Autodesk Inventor part; units mm, degrees
ref_plane "YZ Plane" through (0, 0, 0) normal (1, 0, 0) x (0, 1, 0)
ref_plane "XZ Plane" through (0, 0, 0) normal (0, 1, 0) x (-1, 0, 0)
ref_plane "XY Plane" through (0, 0, 0) normal (0, 0, 1) x (1, 0, 0)
sketch "Sketch1" plane through (0, 0, 0) normal (0, 0, 1) x (1, 0, 0)
  line L0 (2.4705, -2.1641) -> (-67.5295, -2.1641)
  line L1 (-67.5295, -2.1641) -> (-67.5295, 10.5359)
  line L2 (-67.5295, 10.5359) -> (2.4705, 10.5359)
  line L3 (2.4705, 10.5359) -> (2.4705, -2.1641)
  dimension "d0" = 12.7
  dimension "d1" = 70
extrude "Extrusion1" add sketch "Sketch1" along normal blind 567.2
sketch "Sketch2" plane through (2.4705, -2.1641, 0) normal (1, 0, 0) x (0, 0, -1)
  line L0 (-567.3829, 6.35) -> (0, 6.35) construction
  line L1 (0, 12.7) -> (-567.2, 12.7) construction
  line L2 (-567.2, 12.7) -> (-567.2, 0) construction
  point P0 (-543.6, 6.35)
  point P1 (-33.6, 6.35)
  point P2 (-133.6, 6.35)
  point P3 (-238.6, 6.35)
  point P4 (-338.6, 6.35)
  point P5 (-443.6, 6.35)
  dimension "d4" = 6.35
  dimension "d5" = 23.6
  dimension "d6" = 100
  dimension "d7" = 105
  dimension "d8" = 100
  dimension "d9" = 105
  dimension "d10" = 100
  dimension "d11" = 33.6
  dimension "d12" = 567.3829
hole "Hole1" [suppressed]
sketch "Sketch3" plane through (0, 0, 567.2) normal (0, 0, 1) x (1, 0, 0)
  line L0 (-67.5295, -2.1641) -> (-67.5295, 10.5359)
  line L1 (-67.5295, 10.5359) -> (2.4705, 10.5359)
  line L2 (2.4705, -2.1641) -> (-67.5295, -2.1641)
  line L3 (2.4705, 10.5359) -> (2.4705, -2.1641)
extrude "Extrusion2" add sketch "Sketch3" along normal blind 150
sketch "Sketch4" plane through (0, 0, 0) normal (0, 0, -1) x (-1, 0, 0)
  line L0 (-2.4705, -2.1641) -> (67.5295, -2.1641)
  line L1 (67.5295, -2.1641) -> (67.5295, 10.5359)
  line L2 (67.5295, 10.5359) -> (-2.4705, 10.5359)
  line L3 (-2.4705, 10.5359) -> (-2.4705, -2.1641)
extrude "Extrusion3" add sketch "Sketch4" along normal blind 150
sketch "Sketch5" plane through (2.4705, -2.1641, 717.2) normal (1, 0, 0) x (0, 0, -1)
  circle A0 centre (73.972, 6.35) radius 3.9687
  circle A1 centre (113.972, 6.35) radius 3.9687
  circle A2 centre (748.257, 6.35) radius 3.9687
  circle A3 centre (798.257, 6.35) radius 3.9687
hole "Hole2" [suppressed]
sketch "Sketch6" plane through (2.4705, -2.1641, 717.2) normal (1, 0, 0) x (0, 0, -1)
  line L0 (867.2, 0) -> (0, 0)
  line L1 (0, 12.7) -> (0, 0)
  line L2 (0, 12.7) -> (867.2, 12.7)
  line L3 (63.972, 12.7) -> (63.972, 0)
  line L4 (63.972, 12.7) -> (0, 12.7)
  line L5 (0, 0) -> (63.972, 0)
  line L6 (0, 0) -> (0, 12.7)
  circle A0 centre (73.972, 6.35) radius 3.9687
  dimension "d31" = 10
extrude "Extrusion4" cut sketch "Sketch6" against normal blind 70 contours L0 L1 L2 L3
sketch "Sketch7" plane through (2.4705, -2.1641, 653.228) normal (1, 0, 0) x (0, 0, -1)
  line L0 (803.228, 0) -> (0, 0)
  line L1 (0, 12.7) -> (803.228, 12.7)
  line L2 (803.228, 0) -> (803.228, 12.7)
  circle A0 centre (734.285, 6.35) radius 3.9687
  line L3 (749.285, 12.7) -> (749.285, 0)
  line L4 (749.285, 0) -> (803.228, 0)
  line L5 (803.228, 1.1687) -> (803.228, 12.7)
  line L6 (803.228, 12.7) -> (749.285, 12.7)
  dimension "d34" = 15
extrude "Extrusion5" cut sketch "Sketch7" against normal blind 70 contours L0 L3 L1 L2
fillet "Fillet1" radius 3 4 edges at (2.4705, -2.1641, 278.5855) (-32.5295, -2.1641, -96.057) (-67.5295, -2.1641, 278.5855) (-32.5295, -2.1641, 653.228)
fillet "Fillet2" radius 9 4 edges at (-32.5295, 10.5359, 653.228) (-67.5295, 10.5359, 278.5855) (-32.5295, 10.5359, -96.057) (2.4705, 10.5359, 278.5855)
sketch "Sketch8" plane through (-67.5295, 0.8359, 238.6) normal (-1, 0, 0) x (0, 0, 1)
  line L0 (38.016, -32.096) -> (38.016, 13.904)
  line L1 (405.628, 9.7) -> (-325.657, 9.7)
  line L2 (38.016, 3.35) -> (67.7675, 3.35) construction
  line L3 (49.521, 11.9848) -> (49.521, 0.9719) construction
  point P0 (49.521, 3.35)
  dimension "d39" = 11.505
  dimension "d40" = 6.35
hole "Hole3" [suppressed]
sketch "Sketch9" plane through (2.4705, 0.8359, 338.6) normal (1, 0, 0) x (0, 0, -1)
  arc A0 (49.011, 3.658) -> (51.947, 3.658) centre (50.479, 3.35) ccw
hole "Hole4" [suppressed]
ref_plane "Work Plane1" through (-32.5295, -2.1641, 650.228) normal (-1, 0, 0) x (0, 0.9041723, -0.427168)
properties part number "Version 2 field plate"
CAD build for the part. Positions are in the model's coordinates, mm. Give positions to 0.01 mm unless a question says otherwise; leave off trailing zeros. Loops run counter-clockwise (first coordinate to the right, second up) from the corner with the lowest first, then second, coordinate; pieces in that order, holes last. Notation, with made-up numbers: (61.25, -25.75) -> (96.25, -25.75) arc R12 cw to (96.25, -12.75) -> close; hole circle Ø9 at (-4.5, 14.25). An arc over 180 degrees is marked (long way). Use a Markdown table: item, result.
1. Flat gauge pins, fed straight in: pin 1 (3 mm diameter, centred on x = -12, y = 5.5, fed in from +Z); pin 2 (3 mm diameter, centred on y = 8, z = 388.5, fed in from +X). Where does each tip first touch, or does it go through?
Check result:
| item | result |
|---|---|
| pin 1 | stops at z = 652.88 |
| pin 2 | stops at x = 0.98 |
2. Slice it at A-A (z = 428). List the corners of the cut face in (x, y).
Check result:
| item | result |
|---|---|
| outline | (-67.53, 0.84) arc R3 ccw to (-64.53, -2.16) -> (-0.53, -2.16) arc R3 ccw to (2.47, 0.84) -> (2.47, 1.54) arc R9 ccw to (-6.53, 10.54) -> (-58.53, 10.54) arc R9 ccw to (-67.53, 1.54) -> close |
3. Slice it at B-B (y = 7.5). List the corners of the cut face in (x, z), plus the area to 3 significant figures.
Check result:
| item | result |
|---|---|
| outline | (-65.27, -93.8) -> (0.21, -93.8) -> (0.21, 650.97) -> (-65.27, 650.97) -> close |
| area | 48,800 mm^2 |
4. Wall check: L1, parallel to X at y = 2.75, z = 269; L2, parallel to X at y = 8.25, z = -20; L3, parallel to Z at x = -41, y = 2.5. Give the ranges that are in metal, low to high. Write a range as [from, to].
Check result:
| item | result |
|---|---|
| L1 | x = [-67.45, 2.39] |
| L2 | x = [-64.52, -0.54] |
| L3 | z = [-96.01, 653.18] |
